Autodesk Inventor part; units mm, degrees
ref_plane "YZ Plane" through (0, 0, 0) normal (1, 0, 0) x (0, 1, 0)
ref_plane "XZ Plane" through (0, 0, 0) normal (0, 1, 0) x (-1, 0, 0)
ref_plane "XY Plane" through (0, 0, 0) normal (0, 0, 1) x (1, 0, 0)
sketch "Sketch1" plane through (0, 0, 0) normal (0, 0, 1) x (1, 0, 0)
  circle A0 centre (0, 0) radius 15.05
  circle A1 centre (0, 0) radius 24.125
  circle A2 centre (0, 0) radius 25.4
  point P0 (-20, 0)
  point P1 (20, 0)
  dimension "d0" = 30.1
  dimension "d1" = 48.25
  dimension "d2" = 50.8
extrude "Extrusion1" add sketch "Sketch1" along normal blind 5.5 contours A1
extrude "Extrusion2" add sketch "Sketch1" along normal blind 1 contours A2
hole "Hole1" at (-20, 0, 0) at (20, 0, 0) direction (0, 0, 1) diameter 2 end through all
properties part number "Adapter-MitutoyoMT1-SM2"
Design review of the part built by this model. Coordinates are the model's own, in mm. A direction names the side the tool comes from. Round coordinates to 2 decimals unless told otherwise and drop trailing zeros. Write each loop counter-clockwise with the first axis right and the second up, starting at its lowest first coordinate (ties: lowest second). Pieces come first, ordered by that corner, then holes. Notation, with made-up numbers: (-10.75, -37) -> (26.25, -37) arc R9 cw to (26.25, -29) -> close; hole circle Ø7 at (38.5, -14). An arc over 180 degrees is marked (long way). One line per question, with ' | ' between items.
(1) Take a section at A-A, the plane y = 0. State the section outline as (x, z) points (3 decimals), and give its area (3 significant figures).
Result sheet:
outline: (-25.4, 0) -> (-21, 0) -> (-21, 5.5) -> (-24.125, 5.5) -> (-24.125, 1) -> (-25.4, 1) -> close; (-19, 0) -> (-15.05, 0) -> (-15.05, 5.5) -> (-19, 5.5) -> close; (15.05, 0) -> (19, 0) -> (19, 5.5) -> (15.05, 5.5) -> close; (21, 0) -> (25.4, 0) -> (25.4, 1) -> (24.125, 1) -> (24.125, 5.5) -> (21, 5.5) -> close | area: 80.4 mm2
(2) Take a section at B-B, the plane x = 0. State the section outline as (y, z) points (3 decimals).
Result sheet:
outline: (-25.4, 0) -> (-15.05, 0) -> (-15.05, 5.5) -> (-24.125, 5.5) -> (-24.125, 1) -> (-25.4, 1) -> close; (15.05, 0) -> (25.4, 0) -> (25.4, 1) -> (24.125, 1) -> (24.125, 5.5) -> (15.05, 5.5) -> close
(3) Draft analysis for pull direction Y (two halves, no side actions). For faces 1 (the cylindrical face through (-19, 0, 3)), 2 (the cylindrical face through (-24.1, -1.1, 3.2)), 3 (the flat face through (11, -11, 0)), state which applies: released by +Y, released by -Y, zero draft, split by the parting line, or undercut.
Result sheet:
face 1: undercut | face 2: split by the parting line | face 3: zero draft
(4) Wall thickness on line 1 (Y direction, x = 0, z = 2.6) (3 decimals); line 2 (X direction, y = 4.5, z = 4.8); line 3 (X direction, y = 9.5, z = 1.85): over which ranges is each line inside the solid? List them lowest first. Write a range as [from, to].
Result sheet:
line 1: [-24.125, -15.05], [15.05, 24.125] | line 2: [-23.7, -14.36], [14.36, 23.7] | line 3: [-22.18, -11.67], [11.67, 22.18]
(5) Insertion check: P1, Ø1, axis at y = -4, z = 2, coming from the -X side; P2, Ø3, axis at y = 13, z = 3, coming from the -X side; P3, Ø1.2, axis at x = -20, y = 0, coming from the -Z side. Each pin has a flat end and moves straight along its axis. Give the tip position at first contact, or say it passes through.
Result sheet:
P1: x = -23.87 | P2: x = -21.21 | P3: through
(6) Take a section at D-D, the plane z = 4.55. State the section outline as (x, y) points (3 decimals), and give its area (3 significant figures).
Result sheet:
outline: circle Ø48.25 at (0, 0); hole circle Ø2 at (-20, 0); hole circle Ø30.1 at (0, 0); hole circle Ø2 at (20, 0) | area: 1,110 mm2
(7) Machinability: for faces 4 (the flat face through (22.5, -9.3, 1)), 5 (the flat face through (10.4, 11.1, 5.5)), which of the approach directions +Z, -Z, +X, -X, +Y, -Y give a long, thin tool a straight path to every point of the face, cutting with its end or side? Answer none if there is none.
Result sheet:
face 4: +Z | face 5: +Z, +X, -X, +Y, -Y
(8) Take a section at C-C, the plane y = -12. State the section outline as (x, z) points, and give its area (3 significant figures).
Result sheet:
outline: (-22.39, 0) -> (-9.08, 0) -> (-9.08, 5.5) -> (-20.93, 5.5) -> (-20.93, 1) -> (-22.39, 1) -> close; (9.08, 0) -> (22.39, 0) -> (22.39, 1) -> (20.93, 1) -> (20.93, 5.5) -> (9.08, 5.5) -> close | area: 133 mm2
